Geometry check sheet. Reference: the model listing, model coordinates, mm. A direction names the side the tool comes from. Coordinates: 2 decimals unless noted, no trailing zeros. Loops run counter-clockwise (first coordinate to the right, second up) from the corner with the lowest first, then second, coordinate; pieces in that order, holes last. Notation, with made-up numbers: (62.5, 83.5) -> (90.5, 83.5) arc R16 ccw to (90.5, 112.5) -> close; hole circle Ø3 at (-0.75, -10.5). An arc over 180 degrees is marked (long way). Answer as a JSON object with one key per item and string values.
from build123d import *

# Parameters (mm, degrees)
F1_DEPTH  = 25.4
F2_W      = 12.7
F2_H      = 25.4
F3_DEPTH  = 50.8
F4_W      = 12.7
F4_H      = 25.4
F5_DEPTH  = 38.1
F6_DEPTH  = 25.401
F8_DEPTH  = 25.401
F9_R      = 6.35
F10_DEPTH = 76.201


with BuildPart() as f1:
    # F0 (on Front) → F1 (new body, symmetric)
    with BuildSketch(Plane.XZ):
        Polygon((0, 38.1), (0, 0), (76.2, 0), (76.2, 12.7), (50.8, 12.7), (50.8, 25.4), (25.4, 25.4), (25.4, 50.8), (12.7, 50.8), align=None)
        Polygon((0, 50.8), (0, 38.1), (12.7, 50.8), align=None)
    extrude(amount=F1_DEPTH, both=True)

    # F2 (on Top) → F3 (join)
    with BuildSketch(Plane.XY):
        with Locations((31.75, 0)):
            Rectangle(F2_W, F2_H)
    extrude(amount=F3_DEPTH)

    # F4 (on Top) → F5 (join)
    with BuildSketch(Plane.XY):
        with Locations((44.45, 0)):
            Rectangle(F4_W, F4_H)
    extrude(amount=F5_DEPTH)

    # F0 (on Front) → F6 (cut, through all)
    with BuildSketch(Plane.XZ):
        Polygon((0, 50.8), (0, 38.1), (12.7, 50.8), align=None)
    extrude(amount=F6_DEPTH, mode=Mode.SUBTRACT)

    # F7 (on Front) → F8 (cut, through all)
    with BuildSketch(Plane.XZ):
        Polygon((0, 38.1), (12.7, 50.8), (0, 50.8), align=None)
    extrude(amount=-F8_DEPTH, mode=Mode.SUBTRACT)

    # F9 (on Right) → F10 (cut, through all)
    with BuildSketch(Plane.YZ):
        with Locations((0, 12.7)):
            Circle(F9_R)
    extrude(amount=F10_DEPTH, mode=Mode.SUBTRACT)


solid = f1.part
1. Mould release check, pull along Y, two halves, no side actions. Record for faces 1 (the face through (29, -25.4, 20)), 2 (the face through (35, 12.7, 35)), 3 (the face through (29.1, 2.93, 7.066)), 4 (the face through (25.4, 19, 38)): released by +Y, released by -Y, zero draft, split by the parting line, or undercut.
Evaluation:
{"face 1": "released by -Y", "face 2": "released by +Y", "face 3": "undercut", "face 4": "zero draft"}
2. Section check B-B, the plane y = 0. Record the boundary of the cut face in (x, z).
Evaluation:
{"outline": "(0, 0) -> (76.2, 0) -> (76.2, 6.35) -> (0, 6.35) -> close; (0, 19.05) -> (50.8, 19.05) -> (50.8, 38.1) -> (38.1, 38.1) -> (38.1, 50.8) -> (12.7, 50.8) -> (0, 38.1) -> close"}
3. Depth check by flat-ended pin: P1, Ø6.5, axis at y = 18, z = 38.5, coming from the +X side; P2, Ø12.5, axis at x = 42, z = 37.5, coming from the -Y side; P3, Ø21, axis at x = 66, y = -20.5, coming from the +Z side; P4, Ø11.5, axis at y = 0, z = 12.7, coming from the +X side. Enter the tip coordinate at first touch or a pass-through.
Evaluation:
{"P1": "stops at x = 25.4", "P2": "stops at y = -12.7", "P3": "stops at z = 12.7", "P4": "passes through"}
4. Section check C-C, the plane z = 42. Record the boundary of the cut face in (x, y), then the cut area to 3 significant figures.
Evaluation:
{"outline": "(3.9, -25.4) -> (25.4, -25.4) -> (25.4, -12.7) -> (38.1, -12.7) -> (38.1, 12.7) -> (25.4, 12.7) -> (25.4, 25.4) -> (3.9, 25.4) -> close", "area": "1,410 mm^2"}
5. Section check D-D, the plane y = 22.5. Record the boundary of the cut face in (x, z), then the cut area to 3 significant figures.
Evaluation:
{"outline": "(0, 0) -> (76.2, 0) -> (76.2, 12.7) -> (50.8, 12.7) -> (50.8, 25.4) -> (25.4, 25.4) -> (25.4, 50.8) -> (12.7, 50.8) -> (0, 38.1) -> close", "area": "2,180 mm^2"}
6. Tool access check on faces 5 (the face through (25.4, -19, 38)), 6 (the face through (38, 0, 0)), 7 (the face through (50.8, 0, 25)), 8 (the face through (38, 19, 25.4)). Record the directions out of +Z, -Z, +X, -X, +Y, -Y that give a thin tool (end or side, any length) a straight path to the whole face; none if there is none.
Evaluation:
{"face 5": "+Z, +X, -Y", "face 6": "-Z, +X, -X, +Y, -Y", "face 7": "+Z, +X, +Y, -Y", "face 8": "+Z, +X, +Y"}
7. Thickness scan on probe 1 along Z at (x, y) = (38, 0); probe 2 along Y at (x, z) = (29, 12.7); probe 3 along X at (y, z) = (19, 31). Record the ranges inside material, lowest first. Write a range as from..to.
Evaluation:
{"probe 1": "z = 0..6.35, 19.05..50.8", "probe 2": "y = -25.4..-6.35, 6.35..25.4", "probe 3": "x = 0..25.4"}
8. Section check A-A, the plane x = 32.5. Record the boundary of the cut face in (y, z), then the cut area to 3 significant figures.
Evaluation:
{"outline": "(-25.4, 0) -> (25.4, 0) -> (25.4, 25.4) -> (12.7, 25.4) -> (12.7, 50.8) -> (-12.7, 50.8) -> (-12.7, 25.4) -> (-25.4, 25.4) -> close; hole circle Ø12.7 at (0, 12.7)", "area": "1,810 mm^2"}
